Could you check a few things on this model? Use its own coordinates, in mm. Give positions to 0.01 mm unless a question says otherwise; leave off trailing zeros. Order: outer loops, then holes, each group sorted by start corner. A loop starts at its lowest first (then second) coordinate and runs counter-clockwise, first axis right, second up.
(1) Imagine slicing it at A-A, the plane x = 11. Write out the boundary of the cut face in (y, z), then the cut area to 3 significant figures.
(2) If I drill on probe 1 along Y at (x, z) = (-11, 13.5); probe 2 along X at (y, z) = (-44, 51.5); probe 3 along X at (y, z) = (-14.5, 27.5), over which ranges is the centre line in solid material (lowest first)?
(3) Will these pins go through, and if not, where does the flat tip stop? pin 1 (12 mm diameter, centred on x = -22.5, z = 28, fed in from -Y); pin 2 (10 mm diameter, centred on x = 39.5, z = 10, fed in from -Y); pin 3 (1 mm diameter, centred on x = -22, y = -6, fed in from +Z).
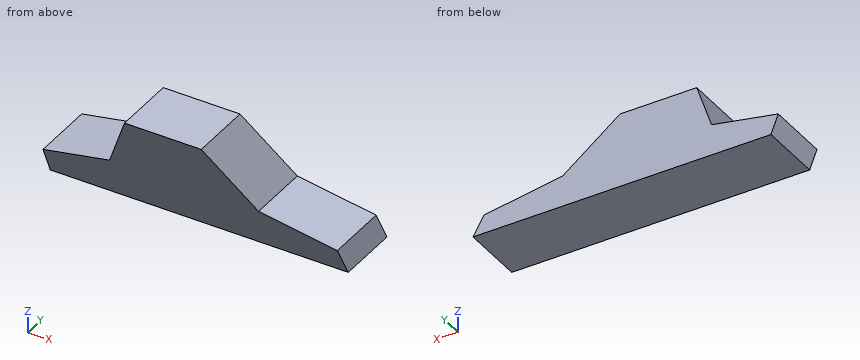
from build123d import *


with BuildPart() as f6:
    # F5 (on plane+point) → F6 section 0
    with BuildSketch(Plane(origin=(0, -22.6192606546, -11.0321505505), x_dir=(-1, 0, 0), z_dir=(0, 0.8987940463, 0.4383711468))):
        Polygon((-66, 12.2743921101), (0, 12.2743921101), (66, 12.2743921101), (65.2149606564, 27.2538351314), (33, 37.2743921101), (17, 72.2743921101), (0, 72.2743921101), (-17, 72.2743921101), (-33, 37.2743921101), (-65.2149606564, 27.2538351314), align=None)
    # F2 (on line) → F6 section 1
    with BuildSketch(Plane(origin=(0, 0, 0), x_dir=(-1, 0, 0), z_dir=(0, 0.8987940463, 0.4383711468))):
        Polygon((-66, 0), (0, 0), (66, 0), (65.2149606564, 14.9794430213), (33, 25), (17, 60), (0, 60), (-17, 60), (-33, 25), (-65.2149606564, 14.9794430213), align=None)
    loft()


solid = f6.part
Answer block:
1. outline: (-54.3, 53.93) - (-28, 0) - (0, 0) - (-26.3, 53.93) - close
1. area: 1,510 mm2
2. probe 1: y = -34.58 to -6.58
2. probe 2: x = -18.23 to 18.23
2. probe 3: x = -30.44 to 30.44
3. pin 1: stops at y = -44.58
3. pin 2: stops at y = -35.32
3. pin 3: stops at z = 13.33
